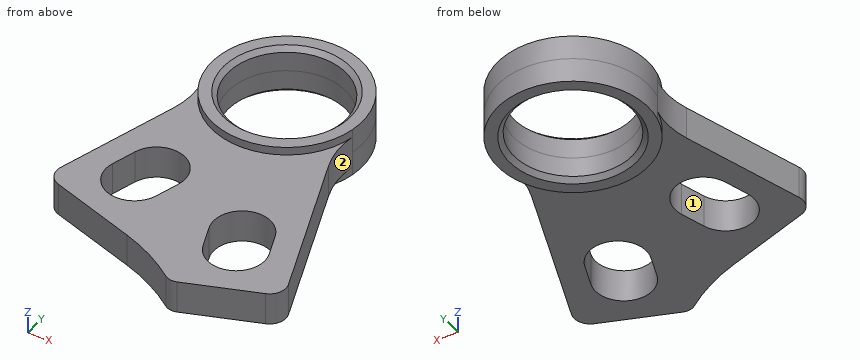
from build123d import *

# Parameters (mm, degrees)
SKETCH1_R           = 11.5062
BOSS_EXTRUDE2_DEPTH = 4.7625
BOSS_EXTRUDE3_DEPTH = 3.175
FILLET1_R           = 3.175
CHAMFER1_SIZE       = 0.889


with BuildPart() as part:
    # Sketch1 → Boss-Extrude2 (new, symmetric)
    with BuildSketch(Plane.XY):
        with BuildLine():
            ThreePointArc((14.454574535, -2.569612511), (-0.50143503, 14.672634268), (-14.245423001, -3.550430532))
            ThreePointArc((-14.245423001, -3.550430532), (0.50143503, -14.672634268), (14.454574535, -2.569612511))
        make_face()
        with Locations(Location((0, 0, 0), (0, 0, 180))):
            Circle(SKETCH1_R, mode=Mode.SUBTRACT)
    extrude(amount=BOSS_EXTRUDE2_DEPTH, both=True)

    # Sketch1_4 → Boss-Extrude3 (add, symmetric)
    with BuildSketch(Plane.XY):
        with BuildLine():
            ThreePointArc((-14.245423001, -3.550430532), (-13.779661889, -7.805545679), (-14.467705296, -12.030416635))
            Line((-14.467705296, -12.030416635), (-22.491098066, -38.27714082))
            Line((-22.491098066, -38.27714082), (-2.755140848, -44.310249384))
            ThreePointArc((-2.755140848, -44.310249384), (3.08819115, -46.639517528), (8.468620942, -49.898504209))
            ThreePointArc((8.468620942, -49.898504209), (9.641965512, -50.366054867), (10.896408583, -50.218699247))
            Line((10.896408583, -50.218699247), (27.771706227, -43.770411636))
            Line((27.771706227, -43.770411636), (15.255266531, -11.014638624))
            ThreePointArc((15.255266531, -11.014638624), (14.280396638, -6.846597475), (14.454574535, -2.569612511))
            ThreePointArc((14.454574535, -2.569612511), (0.50143503, -14.672634268), (-14.245423001, -3.550430532))
        make_face()
        with BuildLine():
            ThreePointArc((-4.293038232, -33.050014953), (-11.230863635, -36.739243436), (-14.920092118, -29.801418033))
            Line((-14.920092118, -29.801418033), (-13.527836296, -25.246966368))
            ThreePointArc((-13.527836296, -25.246966368), (-6.590010893, -21.557737884), (-2.900782409, -28.495563287))
            Line((-2.900782409, -28.495563287), (-4.293038232, -33.050014953))
        make_face(mode=Mode.SUBTRACT)
        with BuildLine():
            ThreePointArc((19.639727055, -35.831335962), (16.432751029, -43.004838098), (9.259248893, -39.797862073))
            Line((9.259248893, -39.797862073), (7.559309131, -35.349085718))
            ThreePointArc((7.559309131, -35.349085718), (10.766285157, -28.175583582), (17.939787293, -31.382559607))
            Line((17.939787293, -31.382559607), (19.639727055, -35.831335962))
        make_face(mode=Mode.SUBTRACT)
    extrude(amount=BOSS_EXTRUDE3_DEPTH, both=True)

    # Fillet1
    fillet1_edges = [part.edges().sort_by_distance(p)[0] for p in [
        (-22.491098066, -38.27714082, 0),
        (27.771706227, -43.770411636, 0),
    ]]
    fillet(fillet1_edges, radius=FILLET1_R)

    # Chamfer1
    chamfer1_edges = [part.edges().sort_by_distance(p)[0] for p in [
        (11.5062, 0, -4.7625),
        (11.5062, 0, 4.7625),
    ]]
    chamfer(chamfer1_edges, length=CHAMFER1_SIZE)


solid = part.part
Can you work these out from the model? Positions are in its coordinate system, mm. Face numbers are marked on the shaded views. A direction names the side the tool comes from. Give positions to 0.01 mm unless a question says otherwise; leave off trailing zeros. Order: outer loops, then holes, each group sorted by start corner. A loop starts at its lowest first (then second) coordinate and runs counter-clockwise, first axis right, second up. Notation, with made-up numbers: M -30,2 L 15,2 A23 cw 15,24 Z; hole C 23,54.25 d9. An arc over 180 degrees is marked long. One line per question, with ' | ' between items.
Item 1: Suppose I cut it at D-D, the plane x = -16. Write out the boundary of the cut face in (y, z) (3 decimals), then the cut area to 3 significant figures.
Answer block:
outline: M -40.261,-3.175 L -17.043,-3.175 L -17.043,3.175 L -40.261,3.175 Z | area: 147 mm2
Item 2: Suppose I cut it at A-A, the plane y = 0. Write out the boundary of the cut face in (x, z), then the cut area to 3 significant figures.
Answer block:
outline: M -14.68,-4.76 L -12.4,-4.76 L -11.51,-3.87 L -11.51,3.87 L -12.4,4.76 L -14.68,4.76 Z; M 11.51,-3.87 L 12.4,-4.76 L 14.68,-4.76 L 14.68,4.76 L 12.4,4.76 L 11.51,3.87 Z | area: 58.9 mm2
Item 3: Suppose I cut it at B-B, the plane x = 0. Write out the boundary of the cut face in (y, z) (1 decimal), then the cut area to 3 significant figures.
Answer block:
outline: M -45.3,-3.2 L -14.7,-3.2 L -14.7,-4.8 L -12.4,-4.8 L -11.5,-3.9 L -11.5,3.9 L -12.4,4.8 L -14.7,4.8 L -14.7,3.2 L -45.3,3.2 Z; M 11.5,-3.9 L 12.4,-4.8 L 14.7,-4.8 L 14.7,4.8 L 12.4,4.8 L 11.5,3.9 Z | area: 253 mm2
Item 4: Suppose I cut it at C-C, the plane z = 1. Give the number of separate pieces and of enclosed holes in the cut face, then the cut area to 3 significant figures.
Answer block:
separate pieces: 1 | enclosed holes: 3 | area: 1,320 mm2
Item 5: For the marked faces 1 and 2, which set-ups out of +Z, -Z, +X, -X, +Y, -Y let a thin tool reach every point of the face, with its end or its side?
Answer block:
face 1: +Z, -Z | face 2: +Z, -Z, +X
Item 6: I'm going to push flat-ended pins straight in: pin 1 Ø3 at (x, z) = (-16.5, 2.5) entering from -Y; pin 2 Ø10 at (x, y) = (20.5, -41) entering from -Z (3 decimals); pin 3 Ø4 at (y, z) = (-4.5, 3.5) entering from +X. Where does each tip first touch, or does it pass through?
Answer block:
pin 1: stops at y = -40.57 | pin 2: stops at z = -3.175 | pin 3: stops at x = 14.47
Item 7: Please list where these lines run through material, in increasing order: L1, parallel to Y at x = -8.5, z = 0.25; L2, parallel to Z at x = -1.5, y = -29 (3 decimals); L3, parallel to Y at x = -12.5, z = -1.25.
Answer block:
L1: y = -42.55 to -36.87, -21.32 to -7.76, 7.76 to 11.97 | L2: z = -3.175 to 3.175 | L3: y = -41.33 to -36.17, -23.34 to 7.7
